Work out the finished part from the listing and answer in its coordinate system (mm). Face numbers are marked on the shaded views. Coordinates: 2 decimals unless noted, no trailing zeros. Loops run counter-clockwise (first coordinate to the right, second up) from the corner with the lowest first, then second, coordinate; pieces in that order, holes last. Notation, with made-up numbers: (-26.5, 69) - (20.5, 69) arc R22 cw to (20.5, 78) - close; hole circle Ø6 at (48.5, -35). An arc over 180 degrees is marked (long way). Write each question's results on one line, items separated by ' | '. Start each with the question number.
1. Find the intervals of material crossed by line 1 along Z through (x, y) = (25.5, -3); line 2 along Z through (x, y) = (-41, 1), in increasing order. Write a range as [from, to].
2. A cutting plane is placed at B-B on z = -40. Determine the outline of the cut face in (x, y), then the cut area to 3 significant figures.
3. A cutting plane is placed at D-D on z = -7. Determine the outline of the cut face in (x, y), then the cut area to 3 significant figures.
4. A cutting plane is placed at C-C on x = -7.5. Determine the outline of the cut face in (y, z), then the cut area to 3 significant figures.
5. Determine the mould class of the marked faces 1 and 2 for opening direction Z: released by +Z, released by -Z, zero draft, split by the parting line, or undercut.
6. Each of these flat-tipped pins is pushed along its axis until it touches: P1, Ø3, axis at x = 0, z = 40, coming from the -Y side; P2, Ø3, axis at x = -1, z = -9, coming from the -Y side; P3, Ø2, axis at y = 0, z = -30, coming from the -X side. Where does it stop, or does it pass through?
7. A cutting plane is placed at A-A on x = 40. Determine the outline of the cut face in (y, z).
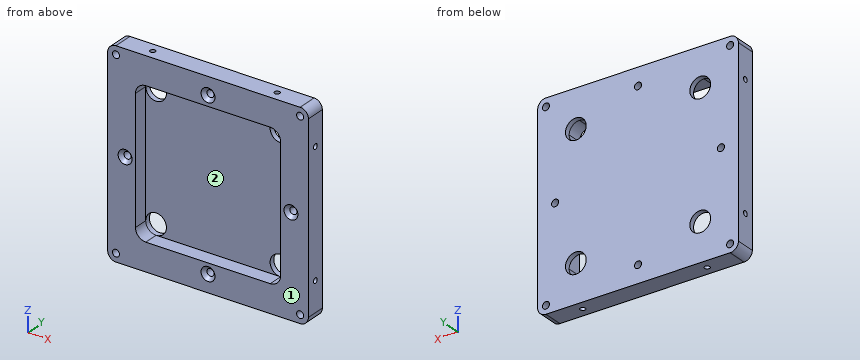
from build123d import *

# Parameters (mm, degrees)
SKETCH1_W                     = 96.825
SKETCH1_H                     = 96.825
BOSS_EXTRUDE1_DEPTH           = 4.7625
FILLET1_R                     = 4
M3X0_5_TAPPED_HOLE1_D         = 2.5
M3X0_5_TAPPED_HOLE1_DEPTH     = 10
M3X0_5_TAPPED_HOLE1_TIP       = 0.751075774
M3X0_5_TAPPED_HOLE2_D         = 2.5
M3X0_5_TAPPED_HOLE2_DEPTH     = 10
M3X0_5_TAPPED_HOLE2_TIP       = 0.751075774
M3_CLEARANCE_HOLE1_D          = 3.4
M3X0_5_TAPPED_HOLE3_D         = 2.5
M3X0_5_TAPPED_HOLE3_DEPTH     = 10
M3X0_5_TAPPED_HOLE3_TIP       = 0.751075774
M3X0_5_TAPPED_HOLE4_D         = 2.5
M3X0_5_TAPPED_HOLE4_DEPTH     = 10
M3X0_5_TAPPED_HOLE4_TIP       = 0.751075774
CSK_FOR_M3_SFHCS1_D           = 3.4
CSK_FOR_M3_SFHCS1_CSINK_D     = 6.72
CSK_FOR_M3_SFHCS1_CSINK_ANGLE = 90
CUT_EXTRUDE1_DEPTH            = 7
SKETCH21_R                    = 5
CUT_EXTRUDE2_DEPTH            = 3.525


with BuildPart() as part:
    # Sketch1 → Boss-Extrude1 (new body, symmetric)
    with BuildSketch(Plane(origin=(0, 0, 0), x_dir=(1, 0, 0), z_dir=(0, 1, 0))):
        Rectangle(SKETCH1_W, SKETCH1_H)
    extrude(amount=BOSS_EXTRUDE1_DEPTH, both=True)

    # Fillet1
    fillet1_edges = [part.edges().sort_by_distance(p)[0] for p in [
        (-48.4125, 0, -48.4125),
        (48.4125, 0, -48.4125),
        (48.4125, 0, 48.4125),
        (-48.4125, 0, 48.4125),
    ]]
    fillet(fillet1_edges, radius=FILLET1_R)

    # M3x0.5 Tapped Hole1
    with Locations(Plane.ZY.offset(48.4125)):
        with Locations((-30, 0), (30, 0)):
            Hole(M3X0_5_TAPPED_HOLE1_D / 2, depth=M3X0_5_TAPPED_HOLE1_DEPTH)
            with Locations((0, 0, -(M3X0_5_TAPPED_HOLE1_DEPTH + M3X0_5_TAPPED_HOLE1_TIP / 2))):  # 118° drill point
                Cone(0, M3X0_5_TAPPED_HOLE1_D / 2, M3X0_5_TAPPED_HOLE1_TIP, mode=Mode.SUBTRACT)

    # M3x0.5 Tapped Hole2
    with Locations(Plane(origin=(0, 0, -48.4125), x_dir=(-1, 0, 0), z_dir=(0, 0, -1))):
        with Locations((-30, 0), (30, 0)):
            Hole(M3X0_5_TAPPED_HOLE2_D / 2, depth=M3X0_5_TAPPED_HOLE2_DEPTH)
            with Locations((0, 0, -(M3X0_5_TAPPED_HOLE2_DEPTH + M3X0_5_TAPPED_HOLE2_TIP / 2))):  # 118° drill point
                Cone(0, M3X0_5_TAPPED_HOLE2_D / 2, M3X0_5_TAPPED_HOLE2_TIP, mode=Mode.SUBTRACT)

    # M3 Clearance Hole1 (through all)
    with Locations(Plane(origin=(0, 4.7625, 0), x_dir=(1, 0, 0), z_dir=(0, 1, 0))):
        with Locations((-44.4125, 44.4125), (44.4125, 44.4125), (44.4125, -44.4125), (-44.4125, -44.4125)):
            Hole(M3_CLEARANCE_HOLE1_D / 2)

    # M3x0.5 Tapped Hole3
    with Locations(Plane(origin=(48.4125, 0, 0), x_dir=(0, 0, -1), z_dir=(1, 0, 0))):
        with Locations((-30, 0), (30, 0)):
            Hole(M3X0_5_TAPPED_HOLE3_D / 2, depth=M3X0_5_TAPPED_HOLE3_DEPTH)
            with Locations((0, 0, -(M3X0_5_TAPPED_HOLE3_DEPTH + M3X0_5_TAPPED_HOLE3_TIP / 2))):  # 118° drill point
                Cone(0, M3X0_5_TAPPED_HOLE3_D / 2, M3X0_5_TAPPED_HOLE3_TIP, mode=Mode.SUBTRACT)

    # M3x0.5 Tapped Hole4
    with Locations(Plane.XY.offset(48.4125)):
        with Locations((-30, 0), (30, 0)):
            Hole(M3X0_5_TAPPED_HOLE4_D / 2, depth=M3X0_5_TAPPED_HOLE4_DEPTH)
            with Locations((0, 0, -(M3X0_5_TAPPED_HOLE4_DEPTH + M3X0_5_TAPPED_HOLE4_TIP / 2))):  # 118° drill point
                Cone(0, M3X0_5_TAPPED_HOLE4_D / 2, M3X0_5_TAPPED_HOLE4_TIP, mode=Mode.SUBTRACT)

    # CSK for M3 SFHCS1 (through all)
    with Locations(Plane(origin=(0, -4.7625, 0), x_dir=(-1, 0, 0), z_dir=(0, -1, 0))):
        with Locations((-40, 0), (0, 40), (40, 0), (0, -40)):
            CounterSinkHole(CSK_FOR_M3_SFHCS1_D / 2, CSK_FOR_M3_SFHCS1_CSINK_D / 2, counter_sink_angle=CSK_FOR_M3_SFHCS1_CSINK_ANGLE)

    # Sketch20 → Cut-Extrude1 (cut)
    with BuildSketch(Plane.XZ.offset(4.7625)):
        with BuildLine():
            Line((30, -35), (-30, -35))
            ThreePointArc((-30, -35), (-33.535533906, -33.535533906), (-35, -30))
            Line((-35, -30), (-35, 30))
            ThreePointArc((-35, 30), (-33.535533906, 33.535533906), (-30, 35))
            Line((-30, 35), (30, 35))
            ThreePointArc((30, 35), (33.535533906, 33.535533906), (35, 30))
            Line((35, 30), (35, -30))
            ThreePointArc((35, -30), (33.535533906, -33.535533906), (30, -35))
        make_face()
    extrude(amount=-CUT_EXTRUDE1_DEPTH, mode=Mode.SUBTRACT)

    # Sketch21 → Cut-Extrude2 (cut, through all)
    with BuildSketch(Plane.XZ.offset(-2.2375)):
        with Locations((-30, 30)):
            Circle(SKETCH21_R)
        with Locations((30, 30)):
            Circle(SKETCH21_R)
        with Locations((30, -30)):
            Circle(SKETCH21_R)
        with Locations((-30, -30)):
            Circle(SKETCH21_R)
    extrude(amount=-CUT_EXTRUDE2_DEPTH, mode=Mode.SUBTRACT)


solid = part.part
Values:
1) line 1: [-48.41, -35], [35, 48.41] | line 2: [-48.41, -30.75], [-29.25, -1.37], [1.37, 29.25], [30.75, 48.41]
2) outline: (-48.41, -4.76) - (-3.36, -4.76) - (-1.7, -3.1) - (-1.7, 4.76) - (-48.41, 4.76) - close; (1.7, -3.1) - (3.36, -4.76) - (48.41, -4.76) - (48.41, 4.76) - (1.7, 4.76) - close; hole circle Ø2.5 at (-30, 0); hole circle Ø2.5 at (30, 0) | area: 877 mm^2
3) outline: (-48.41, -4.76) - (-35, -4.76) - (-35, 2.24) - (35, 2.24) - (35, -4.76) - (48.41, -4.76) - (48.41, 4.76) - (-48.41, 4.76) - close | area: 432 mm^2
4) outline: (-4.76, -48.41) - (4.76, -48.41) - (4.76, 48.41) - (-4.76, 48.41) - (-4.76, 35) - (2.24, 35) - (2.24, -35) - (-4.76, -35) - close | area: 432 mm^2
5) face 1: zero draft | face 2: undercut
6) P1: through | P2: y = 2.24 | P3: x = -38.26
7) outline: (-4.76, -48.41) - (4.76, -48.41) - (4.76, -1.7) - (-3.1, -1.7) - (-4.76, -3.36) - close; (-4.76, 3.36) - (-3.1, 1.7) - (4.76, 1.7) - (4.76, 48.41) - (-4.76, 48.41) - close; hole circle Ø2.5 at (0, -30); hole circle Ø2.5 at (0, 30)
